from build123d import *

# Parameters (mm, degrees)
SKETCH1_W                = 40
SKETCH1_H                = 40
SKETCH1_W_2              = 34
SKETCH1_H_2              = 34
EXTRUDE_THIN1_DEPTH      = 1200
FILLET1_R                = 0.5
FILLET2_R                = 3
F_8_0_8_DIAMETER_HOLE1_D = 8


with BuildPart() as part:
    # Sketch1 → Extrude-Thin1 (new body)
    with BuildSketch(Plane.XY):
        Rectangle(SKETCH1_W, SKETCH1_H)
        Rectangle(SKETCH1_W_2, SKETCH1_H_2, mode=Mode.SUBTRACT)
    extrude(amount=EXTRUDE_THIN1_DEPTH)

    # Fillet1
    fillet1_edges = [part.edges().sort_by_distance(p)[0] for p in [
        (17, -17, 600),
        (17, 17, 600),
        (-17, 17, 600),
        (-17, -17, 600),
    ]]
    fillet(fillet1_edges, radius=FILLET1_R)

    # Fillet2
    fillet2_edges = [part.edges().sort_by_distance(p)[0] for p in [
        (20, -20, 600),
        (-20, -20, 600),
        (-20, 20, 600),
        (20, 20, 600),
    ]]
    fillet(fillet2_edges, radius=FILLET2_R)

    # Ø8.0 (8) Diameter Hole1 (through all)
    with Locations(Plane(origin=(0, 20, 0), x_dir=(1, 0, 0), z_dir=(0, 1, 0))):
        with Locations((0, -20), (0, -1180)):
            Hole(F_8_0_8_DIAMETER_HOLE1_D / 2)


solid = part.part
For this review, take the finished solid that the model builds, in its own axes (mm). A direction names the side the tool comes from. Coordinates: 2 decimals unless noted, no trailing zeros. Loops run counter-clockwise (first coordinate to the right, second up) from the corner with the lowest first, then second, coordinate; pieces in that order, holes last. Notation, with made-up numbers: (-17.75, 46) - (4.25, 46) arc R30 cw to (4.25, 72) - close; hole circle Ø5 at (-7.75, 43). An arc over 180 degrees is marked (long way). Use a Markdown table: item, result. Add a question column.
Item 1: For line 1 (Z direction, x = 0, y = 18.25); line 2 (Y direction, x = -7, z = 473), list the stretches that pass through material, from the lowest coordinate up.
Item 2: Tool access review of faces 4 (the face through (-20, 0, 592)), 5 (the face through (-17, 0, 592)): name each direction out of +Z, -Z, +X, -X, +Y, -Y from which nothing blocks a thin tool from reaching the whole face with its end or side.
Item 3: Mouldability with a two-part tool opening along Y and no side actions: class faces 1 (the face through (-18, 0, 1200)), 2 (the face through (17, 0, 592)), 3 (the face through (0, -20, 592)) as pulls with the +Y half, pulls with the -Y half, needs draft (parallel to the pull), parting line crosses it, or undercut.
Item 4: We need section A-A (y = -2.5). Give the boundary of the cut face in (x, z), and give its area (3 significant figures).
Item 5: We need section B-B (z = 968.5). Give the boundary of the cut face in (x, y), and give its area (3 significant figures).
Results list:
| question | item | result |
|---|---|---|
| 1 | line 1 | z = 0 to 16, 24 to 1176, 1184 to 1200 |
| 1 | line 2 | y = -20 to -17, 17 to 20 |
| 2 | face 4 | +Z, -Z, -X, +Y, -Y |
| 2 | face 5 | +Z, -Z |
| 3 | face 1 | needs draft |
| 3 | face 2 | undercut |
| 3 | face 3 | pulls with the -Y half |
| 4 | outline | (-20, 0) - (-17, 0) - (-17, 1200) - (-20, 1200) - close; (17, 0) - (20, 0) - (20, 1200) - (17, 1200) - close |
| 4 | area | 7,200 mm^2 |
| 5 | outline | (-20, -17) arc R3 ccw to (-17, -20) - (17, -20) arc R3 ccw to (20, -17) - (20, 17) arc R3 ccw to (17, 20) - (-17, 20) arc R3 ccw to (-20, 17) - close; hole (-17, -16.5) arc R0.5 ccw to (-16.5, -17) - (16.5, -17) arc R0.5 ccw to (17, -16.5) - (17, 16.5) arc R0.5 ccw to (16.5, 17) - (-16.5, 17) arc R0.5 ccw to (-17, 16.5) - close |
| 5 | area | 436 mm^2 |
